from build123d import *

# Parameters (mm, degrees)
FILLET1_R = 0.2


with BuildPart() as part:
    # Sketch1 → Revolve1 (revolve)
    with BuildSketch(Plane.XY):
        Polygon((0, 0), (1, 0), (1, 8), (2.5, 8), (2.5, 9), (1, 9), (1, 16), (2.5, 16), (2.5, 17), (1, 17), (1, 25), (0, 25), align=None)
    revolve(axis=Axis((0, 25, 0), (0, -1, 0)))

    # Fillet1
    fillet1_edges = [part.edges().sort_by_distance(p)[0] for p in [
        (-1, 17, 0),
        (-1, 16, 0),
        (-1, 9, 0),
        (-1, 8, 0),
    ]]
    fillet(fillet1_edges, radius=FILLET1_R)


solid = part.part
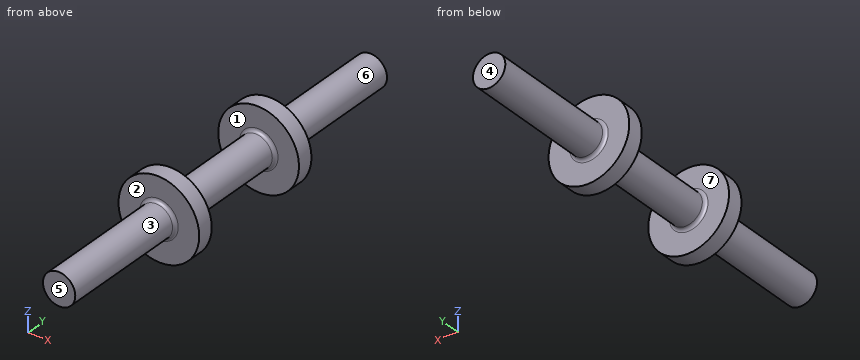
Input: part model. Units: mm. Frame: model coordinates. Face numbers are marked on the shaded views. A direction names the side the tool comes from. Round coordinates to 2 decimals unless told otherwise and drop trailing zeros. Order: outer loops, then holes, each group sorted by start corner. A loop starts at its lowest first (then second) coordinate and runs counter-clockwise, first axis right, second up.
1. Cut plane A-A, the plane z = -2. Output: boundary loops of the cut face in (x, y).
The answers:
outline: (-1.5, 8) - (1.5, 8) - (1.5, 9) - (-1.5, 9) - close; (-1.5, 16) - (1.5, 16) - (1.5, 17) - (-1.5, 17) - close
2. Material intervals for line 1 (Y direction, x = -1.95, z = 0.4); line 2 (Y direction, x = -1, z = -0.35); line 3 (Z direction, x = -0.25, y = 16.5), sorted ascending.
The answers:
line 1: y = 8 to 9, 16 to 17
line 2: y = 7.94 to 9.06, 15.94 to 17.06
line 3: z = -2.49 to 2.49
3. Cut plane B-B, the plane z = 0. Output: boundary loops of the cut face in (x, y).
The answers:
outline: (-2.5, 8) - (-1.2, 8) arc R0.2 cw to (-1, 7.8) - (-1, 0) - (1, 0) - (1, 7.8) arc R0.2 cw to (1.2, 8) - (2.5, 8) - (2.5, 9) - (1.2, 9) arc R0.2 cw to (1, 9.2) - (1, 15.8) arc R0.2 cw to (1.2, 16) - (2.5, 16) - (2.5, 17) - (1.2, 17) arc R0.2 cw to (1, 17.2) - (1, 25) - (-1, 25) - (-1, 17.2) arc R0.2 cw to (-1.2, 17) - (-2.5, 17) - (-2.5, 16) - (-1.2, 16) arc R0.2 cw to (-1, 15.8) - (-1, 9.2) arc R0.2 cw to (-1.2, 9) - (-2.5, 9) - close
4. Cut plane C-C, the plane x = 0. Output: boundary loops of the cut face in (y, z).
The answers:
outline: (0, -1) - (7.8, -1) arc R0.2 cw to (8, -1.2) - (8, -2.5) - (9, -2.5) - (9, -1.2) arc R0.2 cw to (9.2, -1) - (15.8, -1) arc R0.2 cw to (16, -1.2) - (16, -2.5) - (17, -2.5) - (17, -1.2) arc R0.2 cw to (17.2, -1) - (25, -1) - (25, 1) - (17.2, 1) arc R0.2 cw to (17, 1.2) - (17, 2.5) - (16, 2.5) - (16, 1.2) arc R0.2 cw to (15.8, 1) - (9.2, 1) arc R0.2 cw to (9, 1.2) - (9, 2.5) - (8, 2.5) - (8, 1.2) arc R0.2 cw to (7.8, 1) - (0, 1) - close
5. Set-up query: the marked faces 5, 6 and 7. Return all of +Z, -Z, +X, -X, +Y, -Y with unobstructed straight access to the full face (end or side cutting, diameter ignored); none if empty.
The answers:
face 5: +Z, -Z, +X, -X, -Y
face 6: +Y
face 7: none
6. Cut plane D-D, the plane y = 6.75. Output: boundary loops of the cut face in (x, z), then the cut area to 3 significant figures.
The answers:
outline: circle Ø2 at (0, 0)
area: 3.14 mm2
7. Mould query, pull axis Y, two halves, no side actions, for the marked faces 1, 2, 3 and 4. Classes: released by +Y, released by -Y, zero draft, split by the parting line, or undercut.
The answers:
face 1: undercut
face 2: released by -Y
face 3: zero draft
face 4: released by +Y
